from build123d import *

# Parameters (mm, degrees)
SKETCH1_W           = 45
SKETCH1_H           = 25
BOSS_EXTRUDE1_DEPTH = 2.5
SKETCH1_3_R         = 2.5
BOSS_EXTRUDE2_DEPTH = 5
SKETCH2_R           = 1.05
CUT_EXTRUDE1_DEPTH  = 5
SKETCH3_W           = 30.5
SKETCH3_H           = 14.5
CUT_EXTRUDE2_DEPTH  = 2.5


with BuildPart() as part:
    # Sketch1 → Boss-Extrude1 (new body)
    with BuildSketch(Plane.XY):
        with Locations((22.5, 12.5)):
            Rectangle(SKETCH1_W, SKETCH1_H)
    extrude(amount=-BOSS_EXTRUDE1_DEPTH)

    # Sketch1<3> → Boss-Extrude2 (add)
    with BuildSketch(Plane.XY):
        with Locations(Location((3.9, 22, 0), (0, 0, 180))):
            Circle(SKETCH1_3_R)
        with Locations(Location((3.9, 2.5, 0), (0, 0, 270))):
            Circle(SKETCH1_3_R)
        with Locations(Location((41.5, 2.5, 0), (0, 0, 270))):
            Circle(SKETCH1_3_R)
        with Locations(Location((41.5, 22, 0), (0, 0, 180))):
            Circle(SKETCH1_3_R)
    extrude(amount=BOSS_EXTRUDE2_DEPTH)

    # Sketch2 → Cut-Extrude1 (cut)
    with BuildSketch(Plane.XY.offset(5)):
        with Locations((3.9, 22)):
            Circle(SKETCH2_R)
        with Locations((3.9, 2.5)):
            Circle(SKETCH2_R)
        with Locations((41.5, 22)):
            Circle(SKETCH2_R)
        with Locations((41.5, 2.5)):
            Circle(SKETCH2_R)
    extrude(amount=-CUT_EXTRUDE1_DEPTH, mode=Mode.SUBTRACT)

    # Sketch3 → Cut-Extrude2 (cut)
    with BuildSketch(Plane.XY):
        with Locations((23.95, 12.5)):
            Rectangle(SKETCH3_W, SKETCH3_H)
    extrude(amount=-CUT_EXTRUDE2_DEPTH, mode=Mode.SUBTRACT)


solid = part.part
Geometry: final body of the model. Coordinates: model frame, mm. A direction names the side the tool comes from. Coordinates: 2 decimals unless noted, no trailing zeros. Order: outer loops, then holes, each group sorted by start corner. A loop starts at its lowest first (then second) coordinate and runs counter-clockwise, first axis right, second up. Notation, with made-up numbers: (40, 52) - (97, 52) arc R25 ccw to (97, 66) - close; hole circle Ø8 at (1.25, 14). An arc over 180 degrees is marked (long way). Use one line per item in the form item = value.
1) Ray query, L1, parallel to X at y = 2.75, z = 0.75; L2, parallel to X at y = 14.75, z = -1.25; L3, parallel to X at y = 1.75, z = 4.25. Return the intervals inside material, ascending.
Solutions:
L1 = 1.41 to 2.88, 4.92 to 6.39, 39.01 to 40.48, 42.52 to 43.99
L2 = 0 to 8.7, 39.2 to 45
L3 = 1.52 to 3.17, 4.63 to 6.28, 39.12 to 40.77, 42.23 to 43.88
2) Section A-A (z = 1.75). Return loops of the section in (x, y), then the cut area to 3 significant figures.
Solutions:
outline = circle Ø5 at (3.9, 2.5); circle Ø5 at (3.9, 22); circle Ø5 at (41.5, 2.5); circle Ø5 at (41.5, 22); hole circle Ø2.1 at (3.9, 2.5); hole circle Ø2.1 at (3.9, 22); hole circle Ø2.1 at (41.5, 2.5); hole circle Ø2.1 at (41.5, 22)
area = 64.7 mm^2
3) Section D-D (z = -1.25). Return loops of the section in (x, y).
Solutions:
outline = (0, 0) - (45, 0) - (45, 25) - (0, 25) - close; hole (8.7, 5.25) - (39.2, 5.25) - (39.2, 19.75) - (8.7, 19.75) - close
4) Section C-C (y = 13). Return loops of the section in (x, z).
Solutions:
outline = (0, -2.5) - (8.7, -2.5) - (8.7, 0) - (0, 0) - close; (39.2, -2.5) - (45, -2.5) - (45, 0) - (39.2, 0) - close
5) Pin query (flat end, axial travel): pin 1 (10 mm diameter, centred on x = 31, y = 17, fed in from +Z); pin 2 (0.8 mm diameter, centred on y = 15.5, z = -1.5, fed in from -X); pin 3 (1 mm diameter, centred on y = 20, z = 2, fed in from +X). Return the tip coordinate at first contact, or that it passes through.
Solutions:
pin_1 = 0
pin_2 = 0
pin_3 = 43.5
6) Section B-B (x = 37.5). Return loops of the section in (y, z), then the cut area to 4 significant figures.
Solutions:
outline = (0, -2.5) - (5.25, -2.5) - (5.25, 0) - (0, 0) - close; (19.75, -2.5) - (25, -2.5) - (25, 0) - (19.75, 0) - close
area = 26.25 mm^2
7) Mould query, pull axis X, two halves, no side actions, for faces 1 (the face through (40.67, 21.36, 2.54)), 2 (the face through (40, 22, 5)), 3 (the face through (45, 12, -1)), 4 (the face through (41, 22, 0)). Classes: +X half, -X half, draft (parallel to the pull), parting line (faces both ways), or undercut.
Solutions:
face_1 = undercut
face_2 = draft
face_3 = +X half
face_4 = undercut
8) Set-up query: faces 5 (the face through (39.115, 21.249, 2.465)), 6 (the face through (24, 19.75, -1)), 7 (the face through (4, 1, 5)). Return all of +Z, -Z, +X, -X, +Y, -Y with unobstructed straight access to the full face (end or side cutting, diameter ignored); none if empty.
Solutions:
face_5 = +Z
face_6 = +Z, -Z
face_7 = +Z, +X, -X, +Y, -Y
